```python
from build123d import *

# Parameters (mm, degrees)
F1_DEPTH = 30
F3_DEPTH = 30.001
F4_R     = 6


with BuildPart() as f1:
    # F0 (on Top) → F1 (new body)
    with BuildSketch(Plane.XY):
        Polygon((-220, -20), (-220, -50), (220, -50), (220, -20), (50, 60), (-50, 60), align=None)
    extrude(amount=F1_DEPTH)

    # F2 (on face) → F3 (cut, through all)
    with BuildSketch(Plane(origin=(0, 0, 0), x_dir=(1, 0, 0), z_dir=(0, 0, -1))):
        Polygon((-185, 30), (-185, 20.1073184365), (-56.2451380356, -40.4832048408), (-7, 30), align=None)
        Polygon((-1.2777449276, 12), (-40, -43.4220933282), (40, -43.4220933282), (1.2777449276, 12), (0, 13.8288009955), align=None)
        Polygon((185, 30), (7, 30), (56.2451380356, -40.4832048408), (185, 20.1073184365), align=None)
    extrude(amount=-F3_DEPTH, mode=Mode.SUBTRACT)

    # F4
    f4_edges = [f1.edges().sort_by_distance(p)[0] for p in [
        (-185, -20.107318, 15),
        (-185, -30, 15),
        (185, -20.107318, 15),
        (185, -30, 15),
        (-50, 60, 15),
        (50, 60, 15),
        (220, -20, 15),
        (-220, -20, 15),
        (-7, -30, 15),
        (7, -30, 15),
        (0, -13.828801, 15),
        (-56.245138, 40.483205, 15),
        (56.245138, 40.483205, 15),
        (40, 43.422093, 15),
        (-40, 43.422093, 15),
    ]]
    fillet(f4_edges, radius=F4_R)


solid = f1.part
```
Geometry check sheet. Reference: the model listing, model coordinates, mm. A direction names the side the tool comes from. Round coordinates to 2 decimals unless told otherwise and drop trailing zeros. Order: outer loops, then holes, each group sorted by start corner. A loop starts at its lowest first (then second) coordinate and runs counter-clockwise, first axis right, second up. Notation, with made-up numbers: (-23, -38) -> (28, -38) arc R8 ccw to (28, -23) -> close; hole circle Ø10 at (-20, 2.25). An arc over 180 degrees is marked (long way). Return JSON: item names as keys, results as strings. Group by question number.
Q1. Section check C-C, the plane z = 4. Count the separate pieces of the cut face and the enclosed holes in it, plus the area to 3 significant figures.
Q2. Gauge pin test, flat ends, axial feed: pin 1 (10 mm diameter, centred on y = 31.5, z = 17, fed in from +X); pin 2 (8 mm diameter, centred on x = -141.5, z = 9.5, fed in from +Y); pin 3 (9 mm diameter, centred on x = 107, z = 14, fed in from +Y). Record the tip position at first contact, or that the pin passes through.
Q3. Release check for a two-part mould opening along X. For faces 1 (the flat face through (-122.033, 9.524, 14.79)), 2 (the flat face through (-3, -19, 30)), 3 (the flat face through (-220, -37, 15)) record: released by +X, released by -X, zero draft, split by the parting line, or undercut.
Q4. Material ranges on probe 1 along X at (y, z) = (36, 8.5); probe 2 along X at (y, z) = (6, 3); probe 3 along X at (y, z) = (-12.5, 22.5), recorded low to high. Write a range as from..to.
Q5. Section check A-A, the plane y = 2. Record the boundary of the cut face in (x, z).
Q6. Section check B-B, the plane x = 123.5. Record the boundary of the cut face in (y, z), plus the area to 3 significant figures.
Q7. Tool access check on faces 4 (the flat face through (33.2, 7.5, 14.8)), 5 (the flat face through (-3, -19, 0)). Record the directions out of +Z, -Z, +X, -X, +Y, -Y that give a thin tool (end or side, any length) a straight path to the whole face; none if there is none.
Numbers:
{
 "1": {"separate pieces": "1", "enclosed holes": "3", "area": "18,900 mm^2"},
 "2": {"pin 1": "x = 121.19", "pin 2": "y = 18.82", "pin 3": "y = 35.29"},
 "3": {"face 1": "undercut", "face 2": "zero draft", "face 3": "released by -X"},
 "4": {"probe 1": "-101..-65.77, -53.11..-34.32, 34.32..53.11, 65.77..101", "probe 2": "-164.75..-129.52, -32.15..-13.85, 13.85..32.15, 129.52..164.75", "probe 3": "-204.06..-168.83, -19.23..19.23, 168.83..204.06"},
 "5": {"outline": "(-173.25, 0) -> (-138.02, 0) -> (-138.02, 30) -> (-173.25, 30) -> close; (-29.36, 0) -> (-11.06, 0) -> (-11.06, 30) -> (-29.36, 30) -> close; (11.06, 0) -> (29.36, 0) -> (29.36, 30) -> (11.06, 30) -> close; (138.02, 0) -> (173.25, 0) -> (173.25, 30) -> (138.02, 30) -> close"},
 "6": {"outline": "(-50, 0) -> (-30, 0) -> (-30, 30) -> (-50, 30) -> close; (8.83, 0) -> (25.41, 0) -> (25.41, 30) -> (8.83, 30) -> close", "area": "1,100 mm^2"},
 "7": {"face 4": "+Z, -Z", "face 5": "-Z, +X, -X, +Y, -Y"}
}
